Read the model definition and answer for the solid it produces. Units are mm, in the model's axes. A direction names the side the tool comes from. Coordinates: 2 decimals unless noted, no trailing zeros. Write each loop counter-clockwise with the first axis right and the second up, starting at its lowest first coordinate (ties: lowest second). Pieces come first, ordered by that corner, then holes. Notation, with made-up numbers: (52, -4) -> (92, -4) arc R19 cw to (92, 26) -> close; hole circle Ø3 at (-16, -3.5). An arc over 180 degrees is marked (long way). Use CSV: the item, a comma, the result in double quotes. Start each with the question number.
from build123d import *

# Parameters (mm, degrees)
SKETCH3_W           = 78.9
SKETCH3_H           = 32
BOSS_EXTRUDE1_DEPTH = 10
SKETCH3_4_R         = 2.375
CUT_EXTRUDE1_DEPTH  = 8
SKETCH4_W           = 55.14
SKETCH4_H           = 39
BOSS_EXTRUDE2_DEPTH = 6
CUT_EXTRUDE2_REACH  = 66.041
SKETCH9_W           = 78.9
SKETCH9_H           = 10
CUT_EXTRUDE4_DEPTH  = 62.929181295
BOSS_EXTRUDE4_START = -6
SKETCH10_R          = 2.65
BOSS_EXTRUDE4_DEPTH = 6
SKETCH11_W          = 55.305509596
SKETCH11_H          = 8
BOSS_EXTRUDE5_DEPTH = 8
FILLET2_R           = 5
CHAMFER3_SIZE       = 1
CHAMFER4_SIZE       = 0.5


with BuildPart() as part:
    # Sketch3 → Boss-Extrude1 (new body)
    with BuildSketch(Plane(origin=(0, 0, 0), x_dir=(1, 0, 0), z_dir=(0, 1, 0))):
        with Locations((0, 16)):
            Rectangle(SKETCH3_W, SKETCH3_H)
    extrude(amount=BOSS_EXTRUDE1_DEPTH)

    # Sketch3<4> → Cut-Extrude1 (cut)
    with BuildSketch(Plane(origin=(0, 0, 0), x_dir=(1, 0, 0), z_dir=(0, 1, 0))):
        with Locations(Location((-34.45, 9.5, 0), (0, 0, 270))):
            Circle(SKETCH3_4_R)
        with Locations(Location((34.45, 9.5, 0), (0, 0, 270))):
            Circle(SKETCH3_4_R)
        with Locations(Location((-34.45, 25.5, 0), (0, 0, 270))):
            Circle(SKETCH3_4_R)
        with Locations(Location((34.45, 25.5, 0), (0, 0, 270))):
            Circle(SKETCH3_4_R)
    extrude(amount=CUT_EXTRUDE1_DEPTH, mode=Mode.SUBTRACT)

    # Sketch4 → Boss-Extrude2 (add)
    with BuildSketch(Plane.XY):
        with Locations((-0.082754798, -19.5)):
            Rectangle(SKETCH4_W, SKETCH4_H)
    extrude(amount=-BOSS_EXTRUDE2_DEPTH)

    # Sketch6 → Cut-Extrude2 (cut, up to next)
    with BuildSketch(Plane.XY, mode=Mode.PRIVATE) as cut_extrude2_sk1:
        with BuildLine():
            Line((-27.652754798, -39), (27.487245202, -39))
            Line((27.487245202, -39), (27.487245202, -32.795515755))
            ThreePointArc((27.487245202, -32.795515755), (27.113130048, -33.279409344), (26.55063318, -33.039175235))
            ThreePointArc((26.55063318, -33.039175235), (22.840340095, -30.952832292), (19.295797115, -33.309804228))
            ThreePointArc((19.295797115, -33.309804228), (18.842245202, -33.599350759), (18.388693289, -33.309804228))
            ThreePointArc((18.388693289, -33.309804228), (14.135992665, -30.988143783), (10.669672877, -34.373435048))
            ThreePointArc((10.669672877, -34.373435048), (10.313792265, -34.774157145), (9.799721264, -34.622630861))
            ThreePointArc((9.799721264, -34.622630861), (7.44477434, -33.719326103), (5.371236745, -35.155354078))
            ThreePointArc((5.371236745, -35.155354078), (4.951993147, -35.42426536), (4.508475892, -35.197613829))
            ThreePointArc((4.508475892, -35.197613829), (2.60438519, -34.058927341), (0.536516234, -34.862722278))
            ThreePointArc((0.536516234, -34.862722278), (0.021886532, -35.001511273), (-0.325508515, -34.597255418))
            ThreePointArc((-0.325508515, -34.597255418), (-3.632594875, -31.292369955), (-7.755777397, -33.496560058))
            ThreePointArc((-7.755777397, -33.496560058), (-8.207754798, -33.782746053), (-8.659732199, -33.496560058))
            ThreePointArc((-8.659732199, -33.496560058), (-11.896894258, -31.262329464), (-15.446236111, -32.95737429))
            ThreePointArc((-15.446236111, -32.95737429), (-15.968076529, -33.16278259), (-16.352419433, -32.754382635))
            ThreePointArc((-16.352419433, -32.754382635), (-20.981382663, -28.205325535), (-26.701290363, -31.271899679))
            ThreePointArc((-26.701290363, -31.271899679), (-27.262908741, -31.544719865), (-27.652754798, -31.057004673))
            Line((-27.652754798, -31.057004673), (-27.652754798, -39))
        make_face()
    cut_extrude2_tool1 = extrude(cut_extrude2_sk1.sketch, amount=-CUT_EXTRUDE2_REACH, mode=Mode.PRIVATE) & part.part
    add(cut_extrude2_tool1.solids().sort_by_distance((-1.936265, -35.219125, 0))[0], mode=Mode.SUBTRACT)

    # Sketch9 → Cut-Extrude4 (cut, through all)
    with BuildSketch(Plane.XY):
        with Locations((0, 5)):
            Rectangle(SKETCH9_W, SKETCH9_H)
    extrude(amount=-CUT_EXTRUDE4_DEPTH, mode=Mode.SUBTRACT)

    # Sketch10 → Boss-Extrude4 (add)
    # profile 1 of 2: a face of its own
    with BuildSketch(Plane(origin=(0, 0, -6), x_dir=(-1, 0, 0), z_dir=(0, 0, -1)).offset(BOSS_EXTRUDE4_START)):
        with BuildLine():
            Line((-27.487245202, 0), (-39.367245202, 0))
            Line((-39.367245202, 0), (-39.367245202, -39.5))
            Line((-39.367245202, -39.5), (-28.287245202, -39.5))
            Line((-28.287245202, -39.5), (-28.287245202, -33.295515755))
            Line((-28.287245202, -33.295515755), (-26.987245202, -33.295515755))
            ThreePointArc((-26.987245202, -33.295515755), (-27.340798593, -33.149069145), (-27.487245202, -32.795515755))
            Line((-27.487245202, -32.795515755), (-27.487245202, 0))
        make_face()
        with Locations((-34.367245202, -11.75)):
            Circle(SKETCH10_R, mode=Mode.SUBTRACT)
        with Locations((-34.367245202, -27.75)):
            Circle(SKETCH10_R, mode=Mode.SUBTRACT)
    # profile 2 of 2: a face of its own
    with BuildSketch(Plane(origin=(0, 0, -6), x_dir=(-1, 0, 0), z_dir=(0, 0, -1)).offset(BOSS_EXTRUDE4_START)):
        with BuildLine():
            Line((27.652754798, 0), (39.532754798, 0))
            Line((39.532754798, 0), (39.532754798, -39.5))
            Line((39.532754798, -39.5), (28.452754798, -39.5))
            Line((28.452754798, -39.5), (28.452754798, -31.557004673))
            Line((28.452754798, -31.557004673), (27.152754798, -31.557004673))
            ThreePointArc((27.152754798, -31.557004673), (27.506308189, -31.410558063), (27.652754798, -31.057004673))
            Line((27.652754798, -31.057004673), (27.652754798, 0))
        make_face()
        with Locations((34.532754798, -11.75)):
            Circle(SKETCH10_R, mode=Mode.SUBTRACT)
        with Locations((34.532754798, -27.75)):
            Circle(SKETCH10_R, mode=Mode.SUBTRACT)
    extrude(amount=BOSS_EXTRUDE4_DEPTH)

    # Sketch11 → Boss-Extrude5 (add)
    with BuildSketch(Plane.XY):
        with Locations((0, -4)):
            Rectangle(SKETCH11_W, SKETCH11_H)
    extrude(amount=BOSS_EXTRUDE5_DEPTH)

    # Fillet2
    fillet2_edges = [part.edges().sort_by_distance(p)[0] for p in [
        (0, -8, 0),
    ]]
    fillet(fillet2_edges, radius=FILLET2_R)

    # Chamfer3
    chamfer3_edges = [part.edges().sort_by_distance(p)[0] for p in [
        (28.287245202, -39.5, -3),
        (39.367245202, -39.5, -3),
        (39.367245202, 0, -3),
        (39.367245202, -19.75, -6),
        (33.827245202, -39.5, -6),
        (28.287245202, -36.397757877, -6),
        (-39.532754798, 0, -3),
        (-39.532754798, -39.5, -3),
        (-28.452754798, -39.5, -3),
        (-28.452754798, -35.528502336, -6),
        (-33.992754798, -39.5, -6),
        (-39.532754798, -19.75, -6),
        (-0.082754798, 0, -6),
    ]]
    chamfer(chamfer3_edges, length=CHAMFER3_SIZE)

    # Chamfer4
    chamfer4_edges = [part.edges().sort_by_distance(p)[0] for p in [
        (26.734094792, -33.226694221, 0),
        (26.734094792, -33.226694221, -6),
        (27.637245202, -33.295515755, 0),
        (28.137245202, -33.295515755, -6),
        (-27.802754798, -31.557004673, 0),
        (-28.302754798, -31.557004673, -6),
        (-15.968076529, -33.16278259, -6),
        (-11.896894258, -31.262329464, -6),
        (-8.207754798, -33.782746053, -6),
        (-3.632594875, -31.292369955, -6),
        (0.021886532, -35.001511273, -6),
        (2.60438519, -34.058927341, -6),
        (4.951993147, -35.42426536, -6),
        (7.44477434, -33.719326103, -6),
        (10.313792265, -34.774157145, -6),
        (14.135992665, -30.988143783, -6),
        (18.842245202, -33.599350759, -6),
        (22.840340095, -30.952832292, -6),
        (-26.885778679, -31.479761993, -6),
        (-20.981382663, -28.205325535, -6),
        (-15.968076529, -33.16278259, 0),
        (-20.981382663, -28.205325535, 0),
        (-26.885778679, -31.479761993, 0),
        (22.840340095, -30.952832292, 0),
        (18.842245202, -33.599350759, 0),
        (14.135992665, -30.988143783, 0),
        (10.313792265, -34.774157145, 0),
        (7.44477434, -33.719326103, 0),
        (4.951993147, -35.42426536, 0),
        (2.60438519, -34.058927341, 0),
        (0.021886532, -35.001511273, 0),
        (-3.632594875, -31.292369955, 0),
        (-8.207754798, -33.782746053, 0),
        (-11.896894258, -31.262329464, 0),
    ]]
    chamfer(chamfer4_edges, length=CHAMFER4_SIZE - 0.0001)  # a hair under: the kernel refuses the full size


with BuildPart() as body_2:
    # Mirror1: mirrored copy
    add(part.part.mirror(Plane(origin=(39.45, 10, 0), x_dir=(1, 0, 0), z_dir=(0, 0, 1))))


solid = body_2.part
1) Find the intervals of material crossed by line 1 along X through (y, z) = (-12.5, 3.75); line 2 along X through (y, z) = (-34, 2.75); line 3 along X through (y, z) = (-10, 1.5), in increasing order.
2) Which of the six approach directions +Z, -Z, +X, -X, +Y, -Y give full straight-line access (tool end or side, diameter ignored) to faces 1 (the face through (0, -8, -6)), 2 (the face through (27.653, -5, -4)), 3 (the face through (-27.653, -5, -4))?
3) Each of these flat-tipped pins is pushed along its axis until it touches: pin 1 (7 mm diameter, centred on x = 34.37, y = -11.75, fed in from -Z); pin 2 (3.5 mm diameter, centred on x = -7.5, z = -6.5, fed in from -Y); pin 3 (20 mm diameter, centred on x = 13, y = -15, fed in from -Z); pin 4 (3 mm diameter, centred on x = -34.53, y = -27.75, fed in from -Z). Where does it stop, or does it pass through?
4) Section B-B, the plane x = -35 is taken. Give the vertices of the cut face in (y, z), plus the area to 3 significant figures.
5) Section A-A, the plane y = -3 is taken. Give the vertices of the cut face in (x, z).
6) Section C-C, the plane z = 2.5 is taken. Count the separate pieces of the cut face and the enclosed holes in it, plus the area to 3 significant figures.
7) Section D-D, the plane y = -11.75 is taken. Give the vertices of the cut face in (x, z).
8) The mould has two halves that part along Y. Classify faces 4 (the face through (-35.76, -14.1, 2.96)), 5 (the face through (-28, -31.557, 3)), 6 (the face through (0, -24, 0)): pulls with the +Y half, pulls with the -Y half, needs draft (parallel to the pull), parting line crosses it, or undercut.
The answers:
1,line 1,"x = -39.53 to -37.07, -31.99 to 31.83, 36.91 to 39.37"
1,line 2,"x = -39.53 to -28.45, -0.46 to 6.53, 9 to 10.75, 28.29 to 39.37"
1,line 3,"x = -39.53 to -36.52, -32.54 to 32.38, 36.36 to 39.37"
2,face 1,"-Z, +X, -X, -Y"
2,face 2,"-Z, +X, +Y, -Y"
2,face 3,"-Z, -X, +Y, -Y"
3,pin 1,"stops at z = 0"
3,pin 2,"stops at y = -8.01"
3,pin 3,"stops at z = -8"
3,pin 4,"passes through"
4,outline,"(-39.5, 0) -> (-30.36, 0) -> (-30.36, 6) -> (-38.5, 6) -> (-39.5, 5) -> close; (-25.14, 0) -> (-14.36, 0) -> (-14.36, 6) -> (-25.14, 6) -> close; (-9.14, 0) -> (0, 0) -> (0, 5) -> (-1, 6) -> (-9.14, 6) -> close"
4,area,"173 mm^2"
5,outline,"(-39.53, 0) -> (-27.65, 0) -> (-27.65, -8) -> (27.65, -8) -> (27.65, 0) -> (39.37, 0) -> (39.37, 5) -> (38.37, 6) -> (-38.53, 6) -> (-39.53, 5) -> close"
6,separate pieces,"1"
6,enclosed holes,"4"
6,area,"2,600 mm^2"
7,outline,"(-39.53, 0) -> (-37.18, 0) -> (-37.18, 6) -> (-38.53, 6) -> (-39.53, 5) -> close; (-31.88, 0) -> (-27.65, 0) -> (-27.65, -0.16) -> (27.65, -0.16) -> (27.65, 0) -> (31.72, 0) -> (31.72, 6) -> (-31.88, 6) -> close; (37.02, 0) -> (39.37, 0) -> (39.37, 5) -> (38.37, 6) -> (37.02, 6) -> close"
8,face 4,"undercut"
8,face 5,"pulls with the -Y half"
8,face 6,"needs draft"
